Autodesk Inventor part; units mm, degrees
ref_plane "Work Plane1" through (0, 9.5, 32) normal (0, 0, 1) x (1, 0, 0)
ref_plane "YZ Plane" through (0, 0, 0) normal (1, 0, 0) x (0, 1, 0)
ref_plane "XZ Plane" through (0, 0, 0) normal (0, 1, 0) x (-1, 0, 0)
sketch "Sketch1" plane through (0, 0, 0) normal (0, 0, 1) x (1, 0, 0)
  line L0 (19, 0) -> (32, 0)
  line L1 (32, 0) -> (32, 19)
  line L2 (32, 19) -> (24, 19)
  line L3 (24, 19) -> (24, 4)
  line L4 (24, 4) -> (19, 4)
  line L5 (19, 4) -> (19, 0)
  line L6 (0, 0) -> (0, 12.2084)
  dimension "d0" = 48
  dimension "d1" = 15
  dimension "d2" = 4
  dimension "d4" = 8
  dimension "d17" = 38
revolve "Revolution1" add sketch "Sketch1" angle 360 about axis through (0, 0, 0) along (0, 1, 0)
chamfer "Chamfer1" distance 1 angle 45 1 edges at (-32, 0, 0)
chamfer "Chamfer2" distance 1 angle 45 1 edges at (-19, 0, 0)
chamfer "Chamfer3" distance 1 angle 45 1 edges at (-24, 19, 0)
thread "Thread1"
ref_plane "Work Plane1" through (0, 9.5, 32) normal (0, 0, 1) x (1, 0, 0)
sketch "Sketch3" plane through (0, 9.5, 32) normal (0, 0, 1) x (1, 0, 0)
  circle A0 centre (0, 0) radius 2.5
  point P0 (0, -9.5)
  dimension "d18" = 5
extrude "Extrusion1" cut sketch "Sketch3" against normal blind 5
thread "Thread2"
pattern_circular "Circular Pattern1" count 3 over 360 about axis through (0, 9.5, 0) along (0, 1, 0) of "Extrusion1"
properties part number "Oring_M48-2_nut" material "Stainless Steel, 440C"
Work out the finished part from the listing and answer in its coordinate system (mm). A direction names the side the tool comes from. Give positions to 0.01 mm unless a question says otherwise; leave off trailing zeros. Loops run counter-clockwise (first coordinate to the right, second up) from the corner with the lowest first, then second, coordinate; pieces in that order, holes last. Notation, with made-up numbers: (-28, -5.5) -> (0, -5.5) arc R25 cw to (0, 16.5) -> close; hole circle Ø6 at (12, 5). An arc over 180 degrees is marked (long way). Use a Markdown table: item, result. Add a question column.
1. Flat-ended cylindrical pins translate along their axes: pin 1 Ø4 at (x, y) = (-7, 17) entering from +Z; pin 2 Ø4.5 at (x, y) = (0, 9.5) entering from +Z; pin 3 Ø3 at (y, z) = (6.5, 21.5) entering from -X; pin 4 Ø6 at (x, y) = (3, 11) entering from +Z. Find the tip coordinate at first contact, or state that the pin passes through.
2. For faces 4 (the flat face through (-19.1, 19, 16.4)), 5 (the flat face through (0, 10, 27)), 6 (the flat face through (-23.365, 9.535, -13.53)), 7 (the flat face through (18, 4, -7)), determine the directions among +Z, -Z, +X, -X, +Y, -Y from which every point of the face is accessible in a straight line to the end or side of a thin tool.
3. Find the intervals of material crossed by probe 1 along X at (y, z) = (10.75, 0); probe 2 along Y at (x, z) = (0, 30.8), in increasing order.
4. Section B-B on x = 0 is taken. Determine the outline of the cut face in (y, z), and give its area (3 significant figures).
5. Section C-C on y = 2.25 is taken. Determine the outline of the cut face in (x, z).
6. Determine the mould class of faces 1 (the flat face through (23.4, 9.54, -13.47)), 2 (the cylindrical face through (-6.94, 10.13, 31.24)), 3 (the cylindrical face through (-0.54, 7.06, 29.54)) for opening direction Z: released by +Z, released by -Z, zero draft, split by the parting line, or undercut.
7. Section A-A on z = 0 is taken. Determine the outline of the cut face in (x, y).
8. Section D-D on y = 9.5 is taken. Determine the outline of the cut face in (x, z).
Results below:
| question | item | result |
|---|---|---|
| 1 | pin 1 | stops at z = 31.61 |
| 1 | pin 2 | stops at z = 27 |
| 1 | pin 3 | stops at x = -24.98 |
| 1 | pin 4 | stops at z = 32 |
| 2 | face 4 | +Z, -Z, +X, -X, +Y |
| 2 | face 5 | +Z |
| 2 | face 6 | none |
| 2 | face 7 | +Y |
| 3 | probe 1 | x = -32 to -24, 24 to 32 |
| 3 | probe 2 | y = 0 to 7, 12 to 19 |
| 4 | outline | (0, -31) -> (1, -32) -> (19, -32) -> (19, -25) -> (18, -24) -> (4, -24) -> (4, -19) -> (1, -19) -> (0, -20) -> close; (0, 20) -> (1, 19) -> (4, 19) -> (4, 24) -> (18, 24) -> (19, 25) -> (19, 32) -> (12, 32) -> (12, 27) -> (7, 27) -> (7, 32) -> (1, 32) -> (0, 31) -> close |
| 4 | area | 316 mm^2 |
| 5 | outline | circle Ø64 at (0, 0); hole circle Ø38 at (0, 0) |
| 6 | face 1 | undercut |
| 6 | face 2 | split by the parting line |
| 6 | face 3 | zero draft |
| 7 | outline | (-32, 1) -> (-31, 0) -> (-20, 0) -> (-19, 1) -> (-19, 4) -> (-24, 4) -> (-24, 18) -> (-25, 19) -> (-32, 19) -> close; (19, 1) -> (20, 0) -> (31, 0) -> (32, 1) -> (32, 19) -> (25, 19) -> (24, 18) -> (24, 4) -> (19, 4) -> close |
| 8 | outline | (-28.88, -13.79) -> (-24.63, -11.33) -> (-22.13, -15.67) -> (-26.38, -18.12) arc R32 ccw to (26.38, -18.12) -> (22.13, -15.67) -> (24.63, -11.33) -> (28.88, -13.79) arc R32 ccw to (2.5, 31.9) -> (2.5, 27) -> (-2.5, 27) -> (-2.5, 31.9) arc R32 ccw to start; hole circle Ø48 at (0, 0) |
